Read the model definition and answer for the solid it produces. Units are mm, in the model's axes. A direction names the side the tool comes from. Round coordinates to 2 decimals unless told otherwise and drop trailing zeros. Write each loop counter-clockwise with the first axis right and the second up, starting at its lowest first coordinate (ties: lowest second). Pieces come first, ordered by that corner, then holes.
from build123d import *

# Parameters (mm, degrees)
F0_W           = 156
F0_H           = 50
F1_DEPTH       = 87
F2_W           = 32
F2_H           = 65
F3_DEPTH       = 50
F4_W           = 50
F4_H           = 58
F5_DEPTH       = 27
F7_D           = 13
F7_CBORE_D     = 18
F7_CBORE_DEPTH = 10
F9_D           = 13
F9_CSINK_D     = 20
F9_CSINK_ANGLE = 90
F10_R          = 12
F11_R          = 3


with BuildPart() as f1:
    # F0 (on Front) → F1 (new body)
    with BuildSketch(Plane.XZ):
        with Locations((78, 25)):
            Rectangle(F0_W, F0_H)
    extrude(amount=F1_DEPTH)

    # F2 (on face) → F3 (cut, through all)
    with BuildSketch(Plane.XY.offset(50)):
        with Locations((16, -32.5)):
            Rectangle(F2_W, F2_H)
        with Locations((140, -32.5)):
            Rectangle(F2_W, F2_H)
    extrude(amount=-F3_DEPTH, mode=Mode.SUBTRACT)

    # F4 (on face) → F5 (cut)
    with BuildSketch(Plane.XY.offset(50)):
        with Locations((78, -29)):
            Rectangle(F4_W, F4_H)
    extrude(amount=-F5_DEPTH, mode=Mode.SUBTRACT)

    # F7 (through all)
    with Locations(Plane(origin=(0, -65, 0), x_dir=(-1, 0, 0), z_dir=(0, 1, 0))):
        with Locations((-140, 23), (-16, 23)):
            CounterBoreHole(F7_D / 2, F7_CBORE_D / 2, F7_CBORE_DEPTH)

    # F9 (through all)
    with Locations(Plane.XY.offset(23)):
        with Locations((76, -15), (76, -42)):
            CounterSinkHole(F9_D / 2, F9_CSINK_D / 2, counter_sink_angle=F9_CSINK_ANGLE)

    # F10
    f10_edges = [f1.edges().sort_by_distance(p)[0] for p in [
        (156, -76, 50),
        (156, -76, 0),
        (0, -76, 50),
        (0, -76, 0),
        (103, -58, 36.5),
        (53, -58, 36.5),
    ]]
    fillet(f10_edges, radius=F10_R)

    # F11
    f11_edges = [f1.edges().sort_by_distance(p)[0] for p in [
        (78, -87, 50),
        (78, -58, 50),
        (53, -23, 50),
        (103, -23, 50),
        (56.514719, -54.485281, 50),
        (99.485281, -54.485281, 50),
        (124, -32.5, 50),
        (134, -65, 50),
        (124, -65, 25),
        (124, 0, 25),
        (78, 0, 23),
        (53, -23, 23),
        (56.514719, -54.485281, 23),
        (78, 0, 0),
        (32, 0, 25),
        (32, -32.5, 50),
        (78, -87, 0),
        (32, -32.5, 0),
        (113.5, 0, 50),
        (42.5, 0, 50),
        (124, -32.5, 0),
        (0, -87, 25),
        (3.514719, -87, 46.485281),
        (3.514719, -87, 3.514719),
        (152.485281, -87, 46.485281),
        (152.485281, -87, 3.514719),
        (156, -87, 25),
        (134, -65, 0),
        (152.485281, -65, 46.485281),
        (152.485281, -65, 3.514719),
        (156, -65, 25),
        (103, 0, 36.5),
        (103, -23, 23),
        (99.485281, -54.485281, 23),
        (53, 0, 36.5),
        (78, -58, 23),
    ]]
    fillet(f11_edges, radius=F11_R)


solid = f1.part
Q1. Section D-D (z = 5) is taken. State how many separate pieces and enclosed holes the cut face has, then the cut area to 3 significant figures.
Verdict:
separate pieces: 1
enclosed holes: 2
area: 9,040 mm2
Q2. Straight lines are drawn through the part: probe 1 along Y at (x, z) = (76, 7); probe 2 along X at (y, z) = (-34, 43.5); probe 3 along X at (y, z) = (-42, 8). For each, find the intervals that lie inside material, in ascending order.
Verdict:
probe 1: y = -87 to -48.5, -35.5 to -21.5, -8.5 to 0
probe 2: x = 32 to 53, 103 to 124
probe 3: x = 32 to 69.5, 82.5 to 124
Q3. Which of the six approach directions +Z, -Z, +X, -X, +Y, -Y give full straight-line access (tool end or side, diameter ignored) to faces 4 (the cylindrical face through (32.9, -33.57, 49.14)), 5 (the conical face through (76.868, -35.387, 19.67)), 6 (the flat face through (78, -58, 37))?
Verdict:
face 4: +Z, -X, +Y
face 5: +Z
face 6: +Z, +Y
Q4. Determine the mould class of faces 1 (the cylindrical face through (78.31, -0.86, 22.1)), 2 (the cylindrical face through (135.38, -65.9, 0.86)), 3 (the cylindrical face through (0.9, -86.14, 25.18)) for opening direction X: pulls with the +X half, pulls with the -X half, needs draft (parallel to the pull), parting line crosses it, or undercut.
Verdict:
face 1: undercut
face 2: needs draft
face 3: pulls with the -X half
Q5. Section B-B (x = 140) is taken. Determine the outline of the cut face in (y, z), then the cut area to 3 significant figures.
Verdict:
outline: (-87, 3) arc R3 ccw to (-84, 0) - (-68, 0) arc R3 ccw to (-65, 3) - (-65, 14) - (-75, 14) - (-75, 16.5) - (-87, 16.5) - close; (-87, 29.5) - (-75, 29.5) - (-75, 32) - (-65, 32) - (-65, 47) arc R3 ccw to (-68, 50) - (-84, 50) arc R3 ccw to (-87, 47) - close
area: 756 mm2
Q6. Flat-ended cylindrical pins translate along their axes: pin 1 Ø20.5 at (x, z) = (16, 23) entering from -Y; pin 2 Ø6.5 at (x, z) = (84, 41) entering from +Y; pin 3 Ø10.5 at (x, y) = (76, -42) entering from -Z; pin 4 Ø5 at (y, z) = (-59, 45) entering from +X. Find the tip coordinate at first contact, or state that the pin passes through.
Verdict:
pin 1: stops at y = -87
pin 2: stops at y = -58
pin 3: passes through
pin 4: stops at x = 124
Q7. Section A-A (y = -15) is taken. Determine the outline of the cut face in (x, z), then the cut area to 3 significant figures.
Verdict:
outline: (32, 3) arc R3 ccw to (35, 0) - (69.5, 0) - (69.5, 19.5) - (66, 23) - (56, 23) arc R3 cw to (53, 26) - (53, 47) arc R3 ccw to (50, 50) - (35, 50) arc R3 ccw to (32, 47) - close; (82.5, 0) - (121, 0) arc R3 ccw to (124, 3) - (124, 47) arc R3 ccw to (121, 50) - (106, 50) arc R3 ccw to (103, 47) - (103, 26) arc R3 cw to (100, 23) - (86, 23) - (82.5, 19.5) - close
area: 2,930 mm2
Q8. Section C-C (x = 76) is taken. Determine the outline of the cut face in (y, z), then the cut area to 3 significant figures.
Verdict:
outline: (-87, 3) arc R3 ccw to (-84, 0) - (-48.5, 0) - (-48.5, 19.5) - (-52, 23) - (-55, 23) arc R3 cw to (-58, 26) - (-58, 47) arc R3 ccw to (-61, 50) - (-84, 50) arc R3 ccw to (-87, 47) - close; (-35.5, 0) - (-21.5, 0) - (-21.5, 19.5) - (-25, 23) - (-32, 23) - (-35.5, 19.5) - close; (-8.5, 0) - (-3, 0) arc R3 ccw to (0, 3) - (0, 20) arc R3 ccw to (-3, 23) - (-5, 23) - (-8.5, 19.5) - close
area: 2,150 mm2
